```python
from build123d import *

# Parameters (mm, degrees)
SKETCH1_R           = 5
SKETCH1_R_2         = 1.5
SKETCH1_W           = 5
SKETCH1_H           = 5
BOSS_EXTRUDE1_DEPTH = 5
FILLET1_R           = 5


with BuildPart() as part:
    # Sketch1 → Boss-Extrude1 (new body)
    with BuildSketch(Plane.XY):
        Polygon((-90, 110), (-90, -110), (90, -110), (90, 110), (63, 110), (63, 100), (-63, 100), (-63, 110), align=None)
        with Locations((0, -85)):
            Circle(SKETCH1_R, mode=Mode.SUBTRACT)
        with Locations((-75, 102.5)):
            Circle(SKETCH1_R_2, mode=Mode.SUBTRACT)
        with Locations(Location((-75, -102.5, 0), (0, 0, 90))):
            Circle(SKETCH1_R_2, mode=Mode.SUBTRACT)
        with Locations((75, -102.5)):
            Circle(SKETCH1_R_2, mode=Mode.SUBTRACT)
        with Locations(Location((75, 102.5, 0), (0, 0, 180))):
            Circle(SKETCH1_R_2, mode=Mode.SUBTRACT)
        with Locations(Location((82.5, 80, 0), (0, 0, 90))):
            Circle(SKETCH1_R_2, mode=Mode.SUBTRACT)
        with Locations((82.5, -80)):
            Circle(SKETCH1_R_2, mode=Mode.SUBTRACT)
        with Locations(Location((-82.5, 80, 0), (0, 0, 270))):
            Circle(SKETCH1_R_2, mode=Mode.SUBTRACT)
        with Locations(Location((-82.5, -80, 0), (0, 0, 180))):
            Circle(SKETCH1_R_2, mode=Mode.SUBTRACT)
        with BuildLine():
            Line((-70, 90), (70, 90))
            Line((70, 90), (70, 15.612494996))
            Line((70, 15.612494996), (12.5, 15.612494996))
            ThreePointArc((12.5, 15.612494996), (0, -20), (-12.5, 15.612494996))
            Line((-12.5, 15.612494996), (-70, 15.612494996))
            Line((-70, 15.612494996), (-70, 90))
        make_face(mode=Mode.SUBTRACT)
        with Locations((-82.5, 102.5)):
            Rectangle(SKETCH1_W, SKETCH1_H, mode=Mode.SUBTRACT)
        with Locations((-67.5, 102.5)):
            Rectangle(SKETCH1_W, SKETCH1_H, mode=Mode.SUBTRACT)
        with Locations((-82.5, -102.5)):
            Rectangle(SKETCH1_W, SKETCH1_H, mode=Mode.SUBTRACT)
        with Locations((-67.5, -102.5)):
            Rectangle(SKETCH1_W, SKETCH1_H, mode=Mode.SUBTRACT)
        with Locations((82.5, -102.5)):
            Rectangle(SKETCH1_W, SKETCH1_H, mode=Mode.SUBTRACT)
        with Locations((67.5, -102.5)):
            Rectangle(SKETCH1_W, SKETCH1_H, mode=Mode.SUBTRACT)
        with Locations((82.5, 102.5)):
            Rectangle(SKETCH1_W, SKETCH1_H, mode=Mode.SUBTRACT)
        with Locations((67.5, 102.5)):
            Rectangle(SKETCH1_W, SKETCH1_H, mode=Mode.SUBTRACT)
        with Locations((82.5, 87.5)):
            Rectangle(SKETCH1_W, SKETCH1_H, mode=Mode.SUBTRACT)
        with Locations((82.5, 72.5)):
            Rectangle(SKETCH1_W, SKETCH1_H, mode=Mode.SUBTRACT)
        with Locations((82.5, -87.5)):
            Rectangle(SKETCH1_W, SKETCH1_H, mode=Mode.SUBTRACT)
        with Locations((82.5, -72.5)):
            Rectangle(SKETCH1_W, SKETCH1_H, mode=Mode.SUBTRACT)
        with Locations((-82.5, 87.5)):
            Rectangle(SKETCH1_W, SKETCH1_H, mode=Mode.SUBTRACT)
        with Locations((-82.5, 72.5)):
            Rectangle(SKETCH1_W, SKETCH1_H, mode=Mode.SUBTRACT)
        with Locations((-82.5, -87.5)):
            Rectangle(SKETCH1_W, SKETCH1_H, mode=Mode.SUBTRACT)
        with Locations((-82.5, -72.5)):
            Rectangle(SKETCH1_W, SKETCH1_H, mode=Mode.SUBTRACT)
    extrude(amount=BOSS_EXTRUDE1_DEPTH)

    # Fillet1
    fillet1_edges = [part.edges().sort_by_distance(p)[0] for p in [
        (-63, 110, 2.5),
        (63, 110, 2.5),
        (90, 110, 2.5),
        (90, -110, 2.5),
        (-90, -110, 2.5),
        (-90, 110, 2.5),
        (-12.5, 15.612494996, 2.5),
        (12.5, 15.612494996, 2.5),
        (70, 15.612494996, 2.5),
        (70, 90, 2.5),
        (-70, 90, 2.5),
        (-70, 15.612494996, 2.5),
    ]]
    fillet(fillet1_edges, radius=FILLET1_R)


solid = part.part
```
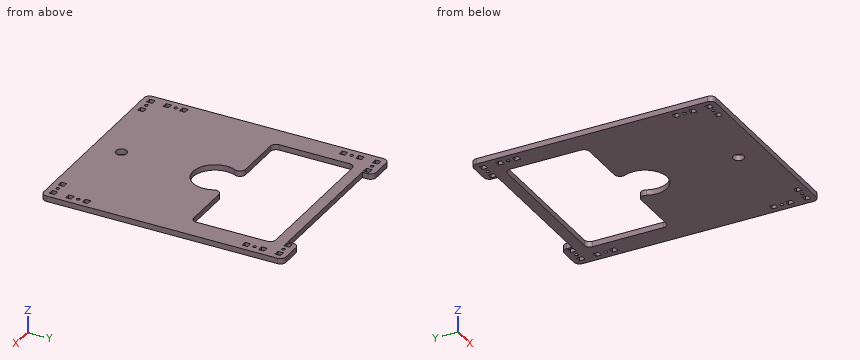
For this review, take the finished solid that the model builds, in its own axes (mm). Coordinates: 2 decimals unless noted, no trailing zeros. Loops run counter-clockwise (first coordinate to the right, second up) from the corner with the lowest first, then second, coordinate; pieces in that order, holes last.
1. Add section A-A, the plane y = 0. Give the boundary of the cut face in (x, z).
2. For line 1 (Y direction, x = -75, z = 2.3); line 2 (X direction, y = -71.5, z = 0.4); line 3 (Y direction, x = 43, z = 1.85), list the stretches that pass through material, from the lowest coordinate up.
3. Add section B-B, the plane x = -10.5. Give the boundary of the cut face in (y, z), then the cut area to 3 significant figures.
4. Add section C-C, the plane z = 3.6. Count the separate pieces of the cut face and the enclosed holes in it, then the cut area to 3 significant figures.
Result:
1. outline: (-90, 0) - (-20, 0) - (-20, 5) - (-90, 5) - close; (20, 0) - (90, 0) - (90, 5) - (20, 5) - close
2. line 1: y = -110 to -104, -101 to 101, 104 to 110
2. line 2: x = -90 to -85, -80 to 80, 85 to 90
2. line 3: y = -110 to 15.61, 90 to 100
3. outline: (-110, 0) - (-17.02, 0) - (-17.02, 5) - (-110, 5) - close; (90, 0) - (100, 0) - (100, 5) - (90, 5) - close
3. area: 515 mm2
4. separate pieces: 1
4. enclosed holes: 26
4. area: 26,200 mm2
